For this review, take the finished solid that the model builds, in its own axes (mm). A direction names the side the tool comes from. Give positions to 0.01 mm unless a question says otherwise; leave off trailing zeros. Write each loop counter-clockwise with the first axis right and the second up, starting at its lowest first coordinate (ties: lowest second). Pieces come first, ordered by that corner, then holes. Notation, with made-up numbers: M 50,54 L 109,54 A27 ccw 109,85 Z; hole C 43.5,88.5 d7. An arc over 180 degrees is marked long. Use one line per item in the form item = value. Start each with the question number.
Q1. Consider section C-C on z = 4. Write out the cut boundary in (x, y), and give its area (3 significant figures).
Q2. Clearance check with flat-ended pins moving along their axes: pin 1 Ø3 at (x, z) = (-7, 1) entering from +Y; pin 2 Ø4 at (x, z) = (-6.5, 6.5) entering from +Y; pin 3 Ø3 at (y, z) = (1.5, 2.5) entering from +X. State where each tip first meets the part, or that it passes through.
Q3. Consider section D-D on z = 6.25. Write out the cut boundary in (x, y).
Q4. Tool access review of faces 4 (the cylindrical face through (1.5, 11.4, 1.1)), 5 (the flat face through (9, -8, 0)): name each direction out of +Z, -Z, +X, -X, +Y, -Y from which nothing blocks a thin tool from reaching the whole face with its end or side.
Q5. Mouldability with a two-part tool opening along X and no side actions: class faces 1 (the cylindrical face through (-14.985, 0.66, 2.416)), 2 (the flat face through (0, 0, 8)), 3 (the flat face through (0, 0, 3)) as released by +X, released by -X, zero draft, split by the parting line, or undercut.
Q6. For probe 1 along Y at (x, z) = (0, 1.4); probe 2 along Z at (x, y) = (-13.5, 8); probe 3 along Z at (x, y) = (10.5, -1), list the stretches that pass through material, from the lowest coordinate up. Write a range as [from, to].
Q7. Consider section A-A on y = 0. Write out the cut boundary in (x, z).
```python
from build123d import *

# Parameters (mm, degrees)
SKETCH3_R           = 15
BOSS_EXTRUDE1_DEPTH = 5
SKETCH4_R           = 11.5
CUT_EXTRUDE1_DEPTH  = 3
FILLET1_R           = 1
FILLET2_R           = 0.2
SKETCH5_R           = 16
BOSS_EXTRUDE2_DEPTH = 3
FILLET3_R           = 0.1


with BuildPart() as part:
    # Sketch3 → Boss-Extrude1 (new body)
    with BuildSketch(Plane.XY):
        Circle(SKETCH3_R)
    extrude(amount=BOSS_EXTRUDE1_DEPTH)

    # Sketch4 → Cut-Extrude1 (cut)
    with BuildSketch(Plane(origin=(0, 0, 0), x_dir=(-1, 0, 0), z_dir=(0, 0, -1))):
        Circle(SKETCH4_R)
    extrude(amount=-CUT_EXTRUDE1_DEPTH, mode=Mode.SUBTRACT)

    # Fillet1
    fillet1_edges = [part.edges().sort_by_distance(p)[0] for p in [
        (11.5, 0, 3),
    ]]
    fillet(fillet1_edges, radius=FILLET1_R)

    # Fillet2
    fillet2_edges = [part.edges().sort_by_distance(p)[0] for p in [
        (11.5, 0, 0),
    ]]
    fillet(fillet2_edges, radius=FILLET2_R)

    # Sketch5 → Boss-Extrude2 (add)
    with BuildSketch(Plane.XY.offset(5)):
        Circle(SKETCH5_R)
    extrude(amount=BOSS_EXTRUDE2_DEPTH)

    # Fillet3
    fillet3_edges = [part.edges().sort_by_distance(p)[0] for p in [
        (-16, 0, 5),
        (-15, 0, 5),
    ]]
    fillet(fillet3_edges, radius=FILLET3_R)


solid = part.part
```
Working result:
q1.outline = C 0,0 d30
q1.area = 707 mm²
q2.pin_1 = 13.96
q2.pin_2 = 15.35
q2.pin_3 = 15
q3.outline = C 0,0 d32
q4.face_4 = -Z
q4.face_5 = -Z, +X, -X, +Y, -Y
q5.face_1 = split by the parting line
q5.face_2 = zero draft
q5.face_3 = undercut
q6.probe_1 = [-15, -11.5], [11.5, 15]
q6.probe_2 = [5, 8]
q6.probe_3 = [3, 8]
q7.outline = M -16,5.1 A0.1 ccw -15.9,5 L -15.1,5 A0.1 cw -15,4.9 L -15,0 L -11.7,0 A0.2 ccw -11.5,0.2 L -11.5,2 A1 cw -10.5,3 L 10.5,3 A1 cw 11.5,2 L 11.5,0.2 A0.2 ccw 11.7,0 L 15,0 L 15,4.9 A0.1 cw 15.1,5 L 15.9,5 A0.1 ccw 16,5.1 L 16,8 L -16,8 Z
